from build123d import *

# Parameters (mm, degrees)
BOSS_EXTRUDE1_DEPTH = 3.175


with BuildPart() as part:
    # Sketch1 → Boss-Extrude1 (new body)
    with BuildSketch(Plane.XY):
        Polygon((0, 0), (29.14, 0), (29.14, 14.24), (29.14, 17.415), (23.312, 17.415), (23.312, 14.24), (11.656, 14.24), (11.656, 17.415), (0, 17.415), (0, 14.24), align=None)
    extrude(amount=BOSS_EXTRUDE1_DEPTH)

    # Mirror1: part across plane


with BuildPart() as part_1:
    add(part.part)
    add(part.part.mirror(Plane(origin=(0, 0, 3.175), x_dir=(0, 0, 1), z_dir=(0, 1, 0))))

    # Mirror3: part across plane


with BuildPart() as part_2:
    add(part_1.part)
    add(part_1.part.mirror(Plane(origin=(29.14, 14.24, 3.175), x_dir=(0, 0, 1), z_dir=(-1, 0, 0))))


solid = part_2.part
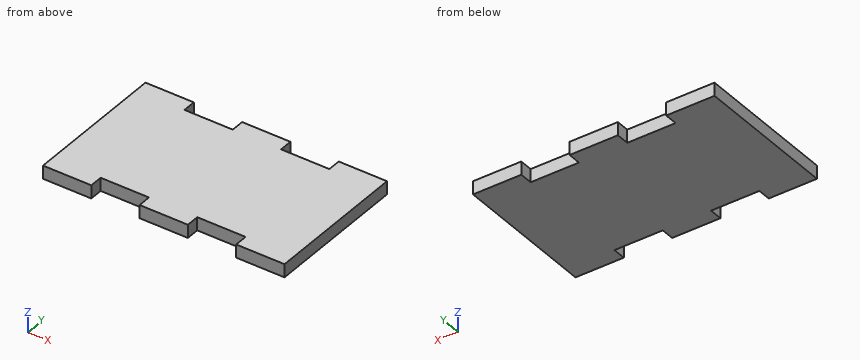
The model under review builds one solid part; all positions refer to its coordinate system, in mm. Give positions to 0.01 mm unless a question says otherwise; leave off trailing zeros. Order: outer loops, then holes, each group sorted by start corner. A loop starts at its lowest first (then second) coordinate and runs counter-clockwise, first axis right, second up. Notation, with made-up numbers: (58, 70) -> (81, 70) arc R21 cw to (81, 106) -> close; hole circle Ø2 at (-21, 73.5). An arc over 180 degrees is marked (long way). Write item = value, one per line. Start each with the question number.
(1) For pin 1 Ø2 at (x, y) = (42.5, 12.5) entering from -Z; pin 2 Ø1.6 at (x, z) = (17, 1) entering from +Y; pin 3 Ø1.6 at (x, z) = (40.5, 2) entering from -Y, all flat-tipped, find the tip position at first contact; note any pin that passes through.
(2) For L1, parallel to X at y = 15, z = 2.75; L2, parallel to Y at x = 19, z = 0.45, list the stretches that pass through material, from the lowest coordinate up. Write a range as from..to.
(3) Take a section at B-B (x = 15). Write out the cut boundary in (y, z) (3 decimals), plus the area to 3 significant figures.
(4) Take a section at A-A (z = 2.1). Write out the cut boundary in (x, y) (3 decimals), plus the area to 3 significant figures.
Returned:
q1.pin_1 = 0
q1.pin_2 = 14.24
q1.pin_3 = -14.24
q2.L1 = 0..11.66, 23.31..34.97, 46.62..58.28
q2.L2 = -14.24..14.24
q3.outline = (-14.24, 0) -> (14.24, 0) -> (14.24, 3.175) -> (-14.24, 3.175) -> close
q3.area = 90.4 mm²
q4.outline = (0, -17.415) -> (11.656, -17.415) -> (11.656, -14.24) -> (23.312, -14.24) -> (23.312, -17.415) -> (34.968, -17.415) -> (34.968, -14.24) -> (46.624, -14.24) -> (46.624, -17.415) -> (58.28, -17.415) -> (58.28, 17.415) -> (46.624, 17.415) -> (46.624, 14.24) -> (34.968, 14.24) -> (34.968, 17.415) -> (23.312, 17.415) -> (23.312, 14.24) -> (11.656, 14.24) -> (11.656, 17.415) -> (0, 17.415) -> close
q4.area = 1,880 mm²
